```python
from build123d import *

# Parameters (mm, degrees)
SKETCH1_W           = 300
SKETCH1_H           = 200
BOSS_EXTRUDE1_DEPTH = 10
BOSS_EXTRUDE2_DEPTH = 300


with BuildPart() as part:
    # Sketch1 → Boss-Extrude1 (new body)
    with BuildSketch(Plane.XY):
        Rectangle(SKETCH1_W, SKETCH1_H)
    extrude(amount=BOSS_EXTRUDE1_DEPTH)

    # Sketch4 → Boss-Extrude2 (add)
    with BuildSketch(Plane(origin=(150, 0, 0), x_dir=(0, 0, -1), z_dir=(1, 0, 0))):
        with BuildLine():
            Line((-10, 78.933179658), (-10, 65.521524353))
            ThreePointArc((-10, 65.521524353), (-27.595666073, 65.410986777), (-36.361743784, 50.15400265))
            Line((-36.361743784, 50.15400265), (-54.176069451, 50.15400265))
            ThreePointArc((-54.176069451, 50.15400265), (-36.361743784, 71.103739422), (-10, 78.933179658))
        make_face()
    extrude(amount=-BOSS_EXTRUDE2_DEPTH)


solid = part.part
```
Work out the finished part from the listing and answer in its coordinate system (mm). A direction names the side the tool comes from. Give positions to 0.01 mm unless a question says otherwise; leave off trailing zeros. Loops run counter-clockwise (first coordinate to the right, second up) from the corner with the lowest first, then second, coordinate; pieces in that order, holes last. Notation, with made-up numbers: (48.25, 19) - (75.25, 19) arc R16 ccw to (75.25, 43) - close; hole circle Ø7 at (64.25, 2). An arc over 180 degrees is marked (long way). One line per question, with ' | ' between items.
(1) Each of these flat-tipped pins is pushed along its axis until it touches: pin 1 Ø5.5 at (x, z) = (5.5, 45.5) entering from -Y; pin 2 Ø6 at (x, z) = (-77, 33) entering from +Y; pin 3 Ø23 at (x, y) = (-56, 85) entering from +Z; pin 4 Ø5 at (x, y) = (-86.5, 63.5) entering from -Z. Where does it stop, or does it pass through?
Recorded:
pin 1: stops at y = 50.15 | pin 2: stops at y = 74.6 | pin 3: stops at z = 32.25 | pin 4: stops at z = 0
(2) A tool of negligible diameter and unlimited length cuts with its end or side. For faces 1 (the face through (2, 50.154, 45)), 2 (the face through (-2, 1, 0)), 3 (the face through (-2, 90, 10)), from which of +Z, -Z, +X, -X, +Y, -Y can it reach the whole face along a straight path? Write none if from no direction.
Recorded:
face 1: +Z, +X, -X, -Y | face 2: -Z, +X, -X, +Y, -Y | face 3: +Z, +X, -X, +Y
(3) The part is cut by section D-D (z = 14). Write down the section's boundary in (x, y), then the cut area to 3 significant figures.
Recorded:
outline: (-150, 67.18) - (150, 67.18) - (150, 78.77) - (-150, 78.77) - close | area: 3,480 mm²
(4) The part is cut by section B-B (x = 128). Write down the section's boundary in (y, z), then the cut area to 3 significant figures.
Recorded:
outline: (-100, 0) - (100, 0) - (100, 10) - (78.93, 10) arc R48.29 ccw to (50.15, 54.18) - (50.15, 36.36) arc R17.66 cw to (65.52, 10) - (-100, 10) - close | area: 2,520 mm²
(5) The part is cut by section A-A (y = 60.5). Write down the section's boundary in (x, z), then the cut area to 3 significant figures.
Recorded:
outline: (-150, 0) - (150, 0) - (150, 10) - (-150, 10) - close; (-150, 33.01) - (150, 33.01) - (150, 47.96) - (-150, 47.96) - close | area: 7,480 mm²
(6) The part is cut by section C-C (y = -29). Write down the section's boundary in (x, z), then the cut area to 3 significant figures.
Recorded:
outline: (-150, 0) - (150, 0) - (150, 10) - (-150, 10) - close | area: 3,000 mm²
(7) Straight lines are drawn through the part: probe 1 along Z at (x, y) = (-116.5, 19.5); probe 2 along Y at (x, z) = (-116, 24); probe 3 along Y at (x, z) = (92.5, 48). For each, find the intervals that lie inside material, in ascending order.
Recorded:
probe 1: z = 0 to 10 | probe 2: y = 67 to 76.86 | probe 3: y = 50.15 to 60.44
